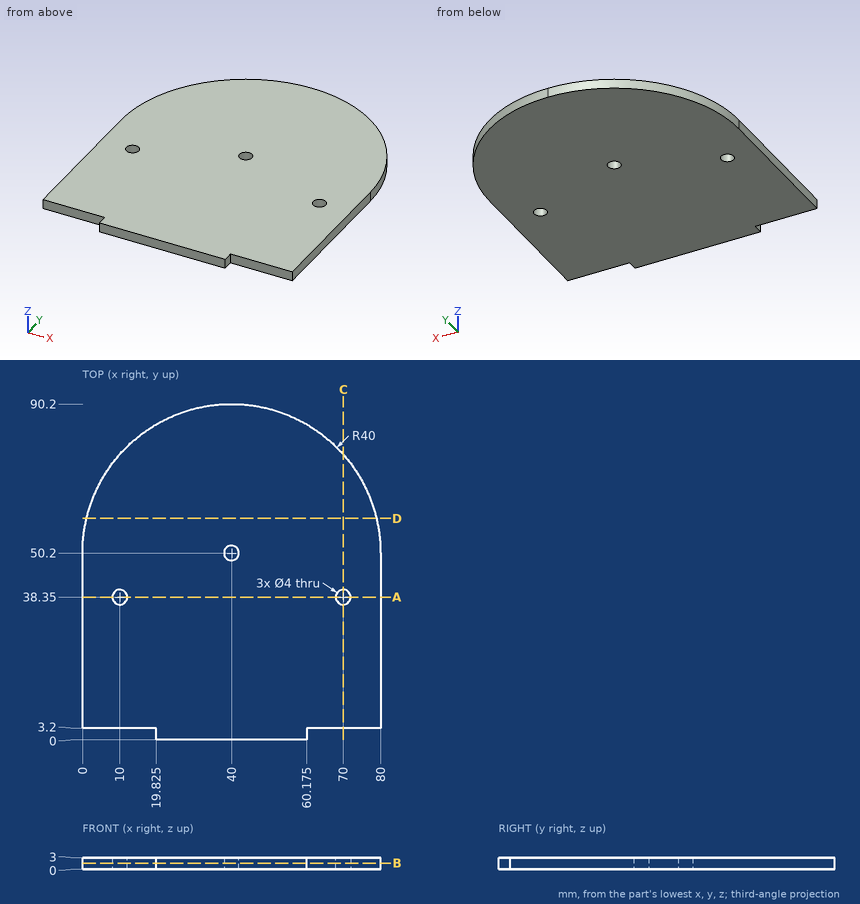
Design review of the part shown in the three views and the two pictorial views. Dimensions are in mm from the part's minimum x, y and z. Round coordinates to 2 decimals unless told otherwise and drop trailing zeros. Order: outer loops, then holes, each group sorted by start corner. A loop starts at its lowest first (then second) coordinate and runs counter-clockwise, first axis right, second up.
Q1. We need section C-C, the plane x = 70. Give the boundary of the cut face in (y, z), plus the area to 3 significant figures.
Findings below:
outline: (3.2, 0) - (36.35, 0) - (36.35, 3) - (3.2, 3) - close; (40.35, 0) - (76.66, 0) - (76.66, 3) - (40.35, 3) - close
area: 208 mm2
Q2. Insertion check: P1, Ø1.5, axis at y = 58.5, z = 2, coming from the +X side; P2, Ø1.5, axis at y = 1.5, z = 1, coming from the +X side (3 decimals); P3, Ø1.5, axis at x = 17.5, z = 2.5, coming from the -Y side. Each pin has a flat end and moves straight along its axis. Give the tip position at first contact, or say it passes through.
Findings below:
P1: stops at x = 79.28
P2: stops at x = 60.175
P3: stops at y = 3.2
Q3. We need section A-A, the plane y = 38.35. Give the boundary of the cut face in (x, z).
Findings below:
outline: (0, 0) - (8, 0) - (8, 3) - (0, 3) - close; (12, 0) - (68, 0) - (68, 3) - (12, 3) - close; (72, 0) - (80, 0) - (80, 3) - (72, 3) - close
Q4. Wall thickness on line 1 (Y direction, x = 40, z = 1.7); line 2 (X direction, y = 51, z = 1.95); line 3 (Y direction, x = 10, z = 1.3): over which ranges is each line inside the solid? List them lowest first.
Findings below:
line 1: y = 0 to 48.2, 52.2 to 90.2
line 2: x = 0.01 to 38.17, 41.83 to 79.99
line 3: y = 3.2 to 36.35, 40.35 to 76.66
Q5. We need section B-B, the plane z = 1.65. Give the boundary of the cut face in (x, y) (3 decimals), plus the area to 3 significant figures.
Findings below:
outline: (0, 3.2) - (19.825, 3.2) - (19.825, 0) - (60.175, 0) - (60.175, 3.2) - (80, 3.2) - (80, 50.2) arc R40 ccw to (0, 50.2) - close; hole circle Ø4 at (10, 38.35); hole circle Ø4 at (40, 50.2); hole circle Ø4 at (70, 38.35)
area: 6,360 mm2
Q6. We need section D-D, the plane y = 59.5. Give the boundary of the cut face in (x, z).
Findings below:
outline: (1.1, 0) - (78.9, 0) - (78.9, 3) - (1.1, 3) - close
